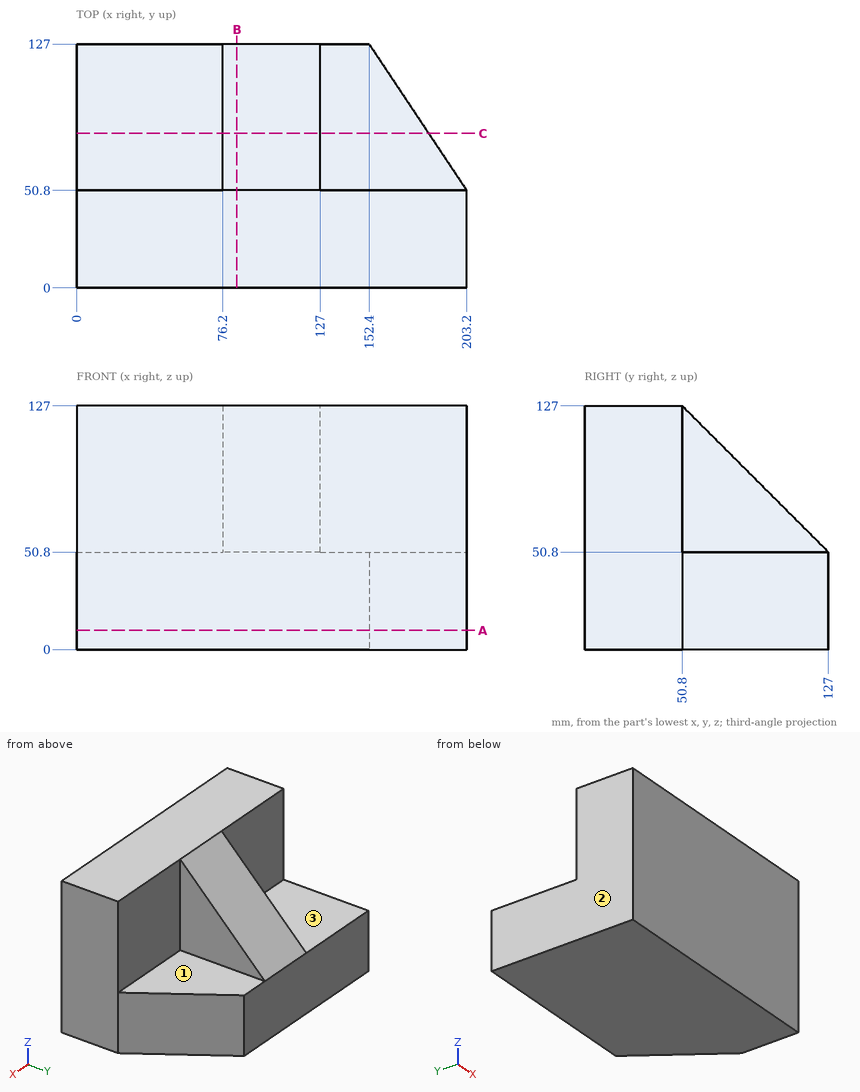
Geometry: see drawing. Coordinates: mm, zero at the bounding-box minimum. A direction names the side the tool comes from. Give positions to 0.01 mm unless a question says otherwise; leave off trailing zeros. Loops run counter-clockwise (first coordinate to the right, second up) from the corner with the lowest first, then second, coordinate; pieces in that order, holes last. Notation, with made-up numbers: (-36.5, 68.5) - (12.5, 68.5) arc R7 cw to (12.5, 78.5) - close; hole circle Ø3 at (12.5, -33.5). An arc over 180 degrees is marked (long way). Answer as CSV lines item,"result". Start each with the question number.
1. Pin query (flat end, axial travel): P1, Ø4, axis at y = 90, z = 63, coming from the +X side; P2, Ø3, axis at y = 77.5, z = 41, coming from the +X side; P3, Ø4, axis at y = 76.5, z = 38.5, coming from the +X side. Return the tip coordinate at first contact, or that it passes through.
2. Section C-C, the plane y = 80.5. Return loops of the section in (x, z), plus the area to 3 significant figures.
3. Section B-B, the plane x = 83.5. Return loops of the section in (y, z), plus the area to 3 significant figures.
4. Section A-A, the plane z = 10. Return loops of the section in (x, y), plus the area to 3 significant figures.
5. Ray query, L1, parallel to Z at x = 182.5, y = 60.5; L2, parallel to X at y = 83.5, z = 75.5. Return the intervals inside material, ascending.
6. Reachability of the marked faces 1, 2 and 3 from +Z, -Z, +X, -X, +Y, -Y: full face, straight path, thin tool, end or side. Return the list, or none.
Answers:
1,P1,"stops at x = 127"
1,P2,"stops at x = 186.4"
1,P3,"stops at x = 187.4"
2,outline,"(0, 0) - (183.4, 0) - (183.4, 50.8) - (127, 50.8) - (127, 97.3) - (76.2, 97.3) - (76.2, 50.8) - (0, 50.8) - close"
2,area,"11,700 mm2"
3,outline,"(0, 0) - (127, 0) - (127, 50.8) - (50.8, 127) - (0, 127) - close"
3,area,"13,200 mm2"
4,outline,"(0, 0) - (203.2, 0) - (203.2, 50.8) - (152.4, 127) - (0, 127) - close"
4,area,"23,900 mm2"
5,L1,"z = 0 to 50.8"
5,L2,"x = 76.2 to 127"
6,face 1,"+Z, +X, +Y"
6,face 2,"+Z, -Z, -X, +Y, -Y"
6,face 3,"+Z, -X, +Y"
